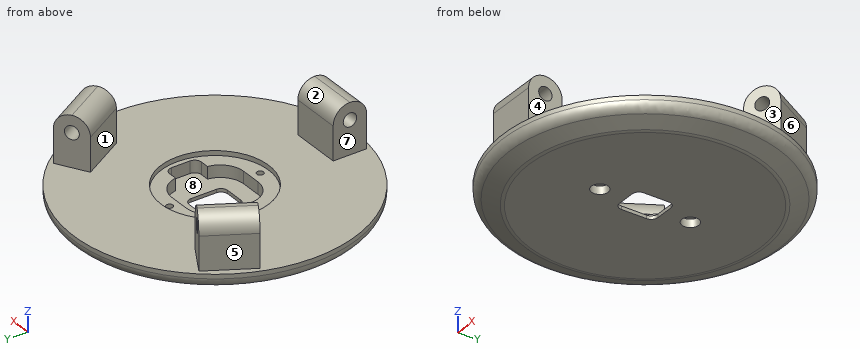
from build123d import *

# Parameters (mm, degrees)
BOSS_EXTRUDE1_DEPTH = 6
SKETCH3_R           = 3
CUT_EXTRUDE1_DEPTH  = 43.330607543
SKETCH8_W           = 20
SKETCH8_H           = 21.4
CUT_EXTRUDE5_DEPTH  = 5
FILLET8_R           = 7
SKETCH9_R           = 1
CUT_EXTRUDE6_DEPTH  = 43.330607543
SKETCH10_W          = 9.5
SKETCH10_H          = 11.5
CUT_EXTRUDE7_DEPTH  = 43.200477899
FILLET9_R           = 2
SKETCH11_W          = 5.5
SKETCH11_H          = 9.5
CUT_EXTRUDE8_DEPTH  = 5
FILLET10_R          = 2
SKETCH12_R          = 16
CUT_EXTRUDE9_DEPTH  = 1.4
SKETCH13_R          = 2.5
CUT_EXTRUDE10_DEPTH = 2.4
SKETCH14_R          = 42
BOSS_EXTRUDE3_DEPTH = 6
CHAMFER1_SIZE       = 2.6
CHAMFER1_SIZE2      = 7.143441291
FILLET12_R          = 3
SKETCH15_W          = 15
SKETCH15_H          = 10
BOSS_EXTRUDE4_DEPTH = 15
SKETCH16_R          = 2
CUT_EXTRUDE11_DEPTH = 15
SKETCH17_R          = 2
CUT_EXTRUDE12_DEPTH = 15
SKETCH18_R          = 2
CUT_EXTRUDE13_DEPTH = 15
FILLET13_R          = 5


with BuildPart() as part:
    # Sketch1 → Boss-Extrude1 (new body)
    with BuildSketch(Plane.XY):
        Polygon((-11.547005384, 20), (-5.63450733, 30.24074703), (5.63450733, 30.24074703), (5.773502692, 30), (23.094010768, 0), (29.006508822, -10.24074703), (23.372001492, -20), (23.094010768, -20), (-11.547005384, -20), (-23.372001492, -20), (-29.006508822, -10.24074703), (-28.867513459, -10), align=None)
    extrude(amount=BOSS_EXTRUDE1_DEPTH)

    # Sketch3 → Cut-Extrude1 (cut, through all)
    with BuildSketch(Plane.XY.offset(6)):
        Circle(SKETCH3_R)
    extrude(amount=-CUT_EXTRUDE1_DEPTH, mode=Mode.SUBTRACT)

    # Sketch8 → Cut-Extrude5 (cut)
    with BuildSketch(Plane.XY.offset(6)):
        Rectangle(SKETCH8_W, SKETCH8_H)
    extrude(amount=-CUT_EXTRUDE5_DEPTH, mode=Mode.SUBTRACT)

    # Fillet8
    fillet8_edges = [part.edges().sort_by_distance(p)[0] for p in [
        (10, 10.7, 3.5),
        (10, -10.7, 3.5),
        (-10, -10.7, 3.5),
        (-10, 10.7, 3.5),
    ]]
    fillet(fillet8_edges, radius=FILLET8_R)

    # Sketch9 → Cut-Extrude6 (cut, through all)
    with BuildSketch(Plane.XY.offset(6)):
        with Locations((0, 13.5)):
            Circle(SKETCH9_R)
        with Locations(Location((0, -13.5, 0), (0, 0, 180))):
            Circle(SKETCH9_R)
    extrude(amount=-CUT_EXTRUDE6_DEPTH, mode=Mode.SUBTRACT)

    # Sketch10 → Cut-Extrude7 (cut, through all)
    with BuildSketch(Plane.XY.offset(1)):
        Rectangle(SKETCH10_W, SKETCH10_H)
    extrude(amount=-CUT_EXTRUDE7_DEPTH, mode=Mode.SUBTRACT)

    # Fillet9
    fillet9_edges = [part.edges().sort_by_distance(p)[0] for p in [
        (4.75, 5.75, 0.5),
        (4.75, -5.75, 0.5),
        (-4.75, -5.75, 0.5),
        (-4.75, 5.75, 0.5),
    ]]
    fillet(fillet9_edges, radius=FILLET9_R)

    # Sketch11 → Cut-Extrude8 (cut)
    with BuildSketch(Plane.XY.offset(6)):
        with Locations((11.75, 0)):
            Rectangle(SKETCH11_W, SKETCH11_H)
    extrude(amount=-CUT_EXTRUDE8_DEPTH, mode=Mode.SUBTRACT)

    # Fillet10
    fillet10_edges = [part.edges().sort_by_distance(p)[0] for p in [
        (14.5, -4.75, 3.5),
        (14.5, 4.75, 3.5),
    ]]
    fillet(fillet10_edges, radius=FILLET10_R)

    # Sketch12 → Cut-Extrude9 (cut)
    with BuildSketch(Plane.XY.offset(6)):
        Circle(SKETCH12_R)
    extrude(amount=-CUT_EXTRUDE9_DEPTH, mode=Mode.SUBTRACT)

    # Sketch13 → Cut-Extrude10 (cut)
    with BuildSketch(Plane(origin=(0, 0, 0), x_dir=(-1, 0, 0), z_dir=(0, 0, -1))):
        with Locations((0, 13.5)):
            Circle(SKETCH13_R)
        with Locations((0, -13.5)):
            Circle(SKETCH13_R)
    extrude(amount=-CUT_EXTRUDE10_DEPTH, mode=Mode.SUBTRACT)

    # Sketch14 → Boss-Extrude3 (add)
    with BuildSketch(Plane(origin=(0, 0, 0), x_dir=(-1, 0, 0), z_dir=(0, 0, -1))):
        Circle(SKETCH14_R)
        Polygon((19.538701505, 0), (9.769350753, 16.921011861), (-9.769350753, 16.921011861), (-19.538701505, 0), (-9.769350753, -16.921011861), (9.769350753, -16.921011861), align=None, mode=Mode.SUBTRACT)
    extrude(amount=-BOSS_EXTRUDE3_DEPTH)

    # Chamfer1
    chamfer1_edges = [part.edges().sort_by_distance(p)[0] for p in [
        (42, 0, 0),
    ]]
    chamfer1_side = [part.faces().sort_by_distance(p)[0] for p in [
        (42, 0, 3),
    ]]
    chamfer(chamfer1_edges, length=CHAMFER1_SIZE, length2=CHAMFER1_SIZE2, reference=chamfer1_side[0])

    # Fillet12
    fillet12_edges = [part.edges().sort_by_distance(p)[0] for p in [
        (34.856558709, 0, 0),
        (42, 0, 2.6),
    ]]
    fillet(fillet12_edges, radius=FILLET12_R)

    # Sketch15 → Boss-Extrude4 (add)
    with BuildSketch(Plane.XY.offset(6)):
        Polygon((-29.730762114, 8.504809472), (-22.230762114, 21.495190528), (-30.891016151, 26.495190528), (-38.391016151, 13.504809472), align=None)
        with Locations((0, -35)):
            Rectangle(SKETCH15_W, SKETCH15_H)
        Polygon((22.230762114, 21.495190528), (29.730762114, 8.504809472), (38.391016151, 13.504809472), (30.891016151, 26.495190528), align=None)
    extrude(amount=BOSS_EXTRUDE4_DEPTH)

    # Sketch16 → Cut-Extrude11 (cut)
    with BuildSketch(Plane(origin=(-3.75, 6.495190528, 0), x_dir=(0.8660254037844431, 0.49999999999999234, 0), z_dir=(-0.4999999999999924, 0.8660254037844431, 0))):
        with Locations(Location((35, -16, 0), (0, 0, 180))):
            Circle(SKETCH16_R)
    extrude(amount=-CUT_EXTRUDE11_DEPTH, mode=Mode.SUBTRACT)

    # Sketch17 → Cut-Extrude12 (cut)
    with BuildSketch(Plane(origin=(7.5, 0, 0), x_dir=(0, 0, -1), z_dir=(1, 0, 0))):
        with Locations(Location((-16, -35, 0), (0, 0, 90))):
            Circle(SKETCH17_R)
    extrude(amount=-CUT_EXTRUDE12_DEPTH, mode=Mode.SUBTRACT)

    # Sketch18 → Cut-Extrude13 (cut)
    with BuildSketch(Plane(origin=(3.75, 6.495190528, 0), x_dir=(0.8660254037844364, -0.5000000000000041, 0), z_dir=(0.500000000000004, 0.8660254037844363, 0))):
        with Locations(Location((-35, -16, 0), (0, 0, 180))):
            Circle(SKETCH18_R)
    extrude(amount=-CUT_EXTRUDE13_DEPTH, mode=Mode.SUBTRACT)

    # Fillet13
    fillet13_edges = [part.edges().sort_by_distance(p)[0] for p in [
        (0, -40, 21),
        (0, -30, 21),
        (-34.641016151, 20, 21),
        (-25.980762114, 15, 21),
        (25.980762114, 15, 21),
        (34.641016151, 20, 21),
    ]]
    fillet(fillet13_edges, radius=FILLET13_R - 0.0001)  # a hair under: the kernel refuses the full size


solid = part.part
Geometry check sheet. Reference: the model listing, model coordinates, mm. Face numbers are marked on the shaded views. A direction names the side the tool comes from. Give positions to 0.01 mm unless a question says otherwise; leave off trailing zeros. Order: outer loops, then holes, each group sorted by start corner. A loop starts at its lowest first (then second) coordinate and runs counter-clockwise, first axis right, second up.
1. Depth check by flat-ended pin: pin 1 (6 mm diameter, centred on x = 0, y = -13.5, fed in from -Z); pin 2 (8 mm diameter, centred on y = -29, z = 3.5, fed in from -X); pin 3 (1.1 mm diameter, centred on y = 1.5, z = 3.5, fed in from +X); pin 4 (3 mm diameter, centred on x = 0.5, z = 2, fed in from -Y). Enter the tip coordinate at first touch or a pass-through.
Completed:
pin 1: stops at z = 0
pin 2: stops at x = -33.66
pin 3: stops at x = 41.9
pin 4: stops at y = -41.75
2. Sectioned sample at B-B (y = 18.5). State how many separate pieces and enclosed holes the cut face has, then the cut area to 3 significant figures.
Completed:
separate pieces: 1
enclosed holes: 2
area: 722 mm2
3. Draft check along X on the marked faces 1, 2 and 3. Enter one of: pulls with the +X half, pulls with the -X half, needs draft (parallel to the pull), parting line crosses it, or undercut.
Completed:
face 1: undercut
face 2: needs draft
face 3: pulls with the +X half
4. Sectioned sample at A-A (z = 9). Record the boundary of the cut face in (x, y).
Completed:
outline: (-38.39, 13.5) - (-29.73, 8.5) - (-22.23, 21.5) - (-30.89, 26.5) - close; (-7.5, -40) - (7.5, -40) - (7.5, -30) - (-7.5, -30) - close; (22.23, 21.5) - (29.73, 8.5) - (38.39, 13.5) - (30.89, 26.5) - close
5. Access from +Z, -Z, +X, -X, +Y, -Y to the whole of each face (thin tool, end or side, straight path). Record for the marked faces 4, 5, 6, 7 and 8.
Completed:
face 4: +Z, +X, +Y, -Y
face 5: +Z, -X, +Y
face 6: +Z, +X, +Y
face 7: +Z, -X, +Y, -Y
face 8: +Z
6. Scan lines: line 1 (Z direction, x = 23, y = -18.5); line 2 (X direction, y = 22, z = 19); line 3 (Y direction, x = 0, z = 3.6). Record each from-to range of solid material in increasing order.
Completed:
line 1: z = 0 to 6
line 2: x = -32.33 to -23.11, 23.11 to 32.33
line 3: y = -41.79 to -14.5, -12.5 to -10.7, 10.7 to 12.5, 14.5 to 41.79
